```python
from build123d import *


with BuildPart() as part:
    # Sketch1 → Revolve2 (revolve)
    with BuildSketch(Plane.XY, mode=Mode.PRIVATE) as revolve2_sk:
        Polygon((0, 0), (0, 6.35), (-3.81, 6.35), (-3.81, 2.794), (-14.986, 2.794), (-14.986, 0), align=None)
    revolve(revolve2_sk.sketch.rotate(Axis((-1364.978742306, 0, 0), (1, 0, 0)), 90), axis=Axis((-1364.978742306, 0, 0), (1, 0, 0)))

    # Sketch4 → Cut-Revolve1 (revolve, cut)
    with BuildSketch(Plane.XY, mode=Mode.PRIVATE) as cut_revolve1_sk:
        Polygon((0, 0), (0, 1.5875), (-2.54, 1.5875), (-3.493866233, 0), align=None)
    revolve(cut_revolve1_sk.sketch.rotate(Axis((0, 0, 0), (-1, 0, 0)), 90), axis=Axis((0, 0, 0), (-1, 0, 0)), mode=Mode.SUBTRACT)


solid = part.part
```
Input: part model. Units: mm. Frame: model coordinates. A direction names the side the tool comes from. Round coordinates to 2 decimals unless told otherwise and drop trailing zeros. Loops run counter-clockwise (first coordinate to the right, second up) from the corner with the lowest first, then second, coordinate; pieces in that order, holes last. Notation, with made-up numbers: M 53,69 L 89,69 A26 cw 89,90 Z; hole C -34.75,0.25 d7. An arc over 180 degrees is marked long. Answer in a Markdown table with one row per item. Add a question column.
1. Set-up query: faces 1 (the face through (-3.81, 1, 3)), 2 (the face through (-1.93, 3.86, -5.04)), 3 (the face through (-1.288, 0.966, 1.26)). Return all of +Z, -Z, +X, -X, +Y, -Y with unobstructed straight access to the full face (end or side cutting, diameter ignored); none if empty.
2. Mould query, pull axis Y, two halves, no side actions, for faces 4 (the face through (0, 1.3, -1.3)), 5 (the face through (-3.34, 0.25, 0.05)), 6 (the face through (-9.476, 1.7, -2.217)). Classes: released by +Y, released by -Y, zero draft, split by the parting line, or undercut.
3. Ray query, probe 1 along Y at (x, z) = (-1.15, 0); probe 2 along X at (y, z) = (0.75, -5.25); probe 3 along Y at (x, z) = (-7.5, 0). Return the intervals inside material, ascending.
4. Section B-B (y = 2). Output: boundary loops of the cut face in (x, z).
5. Section C-C (x = -5.25). Output: boundary loops of the cut face in (y, z).
6. Section D-D (z = -3.75). Output: boundary loops of the cut face in (x, y), and give its area (3 significant figures).
7. Contact query for flat-ended pins moving along their axis: pin 1 (4 mm diameter, centred on x = -8, z = -3.5, fed in from +Y); pin 2 (2 mm diameter, centred on y = 4.5, z = 0, fed in from -X); pin 3 (2 mm diameter, centred on x = -8.5, z = 0.5, fed in from -Y). Output: stop coordinate, or through.
Values follow:
| question | item | result |
|---|---|---|
| 1 | face 1 | -X |
| 1 | face 2 | +X, -X |
| 1 | face 3 | +X |
| 2 | face 4 | zero draft |
| 2 | face 5 | undercut |
| 2 | face 6 | split by the parting line |
| 3 | probe 1 | -6.35 to -1.59, 1.59 to 6.35 |
| 3 | probe 2 | -3.81 to 0 |
| 3 | probe 3 | -2.79 to 2.79 |
| 4 | outline | M -14.99,-1.95 L -3.81,-1.95 L -3.81,-6.03 L 0,-6.03 L 0,6.03 L -3.81,6.03 L -3.81,1.95 L -14.99,1.95 Z |
| 5 | outline | C 0,0 d5.59 |
| 6 | outline | M -3.81,-5.12 L 0,-5.12 L 0,5.12 L -3.81,5.12 Z |
| 6 | area | 39.0 mm^2 |
| 7 | pin 1 | y = 2.36 |
| 7 | pin 2 | x = -3.81 |
| 7 | pin 3 | y = -2.79 |
